from build123d import *

# Parameters (mm, degrees)
F0_W         = 15
F0_H         = 12
F0_R         = 2.5
F1_DEPTH     = 5
F2_R         = 1.5
F3_DEPTH     = 12.001
F4_R         = 0.49999
F5_T1_DEPTH  = 9.5
F5_T3_DEPTH  = 11
F5_T5_DEPTH  = 14
F5_T8_ANGLE  = 90
F5_T10_ANGLE = 90
F5_T12_ANGLE = 90
F5_T14_ANGLE = 90
F5_S17_W     = 0.5
F5_S17_H     = 0.5
F5_T18_DEPTH = 0.5
F5_S23_W     = 0.5
F5_S23_H     = 0.5
F5_T24_DEPTH = 0.5
F5_S29_W     = 0.5
F5_S29_H     = 0.5
F5_T30_DEPTH = 0.5
F5_S35_W     = 0.5
F5_S35_H     = 0.5
F5_T36_DEPTH = 0.5


# Not quite as in the source:
# - a fillet or chamfer that OpenCascade refuses, or shapes differently, is made with other operations: its cross-section is extruded or revolved along the edge and cut away or added
# - a fillet or chamfer is up to 0.001 mm smaller than in the source, because OpenCascade refuses the exact size


with BuildPart() as f1:
    # F0 (on Top) → F1 (new body, symmetric)
    with BuildSketch(Plane.XY):
        with Locations((7.5, 6)):
            Rectangle(F0_W, F0_H)
        with Locations((4.5, 5.5)):
            Circle(F0_R, mode=Mode.SUBTRACT)
    extrude(amount=F1_DEPTH, both=True)

    # F2 (on face) → F3 (cut, through all)
    with BuildSketch(Plane.XZ):
        with Locations((11, 3)):
            Circle(F2_R)
    extrude(amount=-F3_DEPTH, mode=Mode.SUBTRACT)

    # F4 (radius 0.5 in the source; OpenCascade refuses exactly that, so slightly less here)
    f4_edges = [f1.edges().sort_by_distance(p)[0] for p in [
        (7.5, 0, 5),
        (15, 6, 5),
        (7.5, 12, 5),
        (0, 6, 5),
    ]]
    fillet(f4_edges, radius=F4_R)

    # F5: fillet of radius 0.5 on 8 edges, made by hand

    # F5_s2 → F5_t1 (cut)
    with BuildSketch(Plane.XY.offset(-4.5)):
        with BuildLine():
            ThreePointArc((14.5, 0), (14.8535533906, 0.1464466094), (15, 0.5))
            Line((15, 0.5), (15, 0))
            Line((15, 0), (14.5, 0))
        make_face()
        with BuildLine():
            ThreePointArc((0, 0.5), (0.1464466094, 0.1464466094), (0.5, 0))
            Line((0.5, 0), (0, 0))
            Line((0, 0), (0, 0.5))
        make_face()
        with BuildLine():
            ThreePointArc((0, 11.5), (0.1464466094, 11.8535533906), (0.5, 12))
            Line((0.5, 12), (0, 12))
            Line((0, 12), (0, 11.5))
        make_face()
        with BuildLine():
            ThreePointArc((14.5, 12), (14.8535533906, 11.8535533906), (15, 11.5))
            Line((15, 11.5), (15, 12))
            Line((15, 12), (14.5, 12))
        make_face()
    extrude(amount=F5_T1_DEPTH, mode=Mode.SUBTRACT)

    # F5_s4 → F5_t3 (cut)
    with BuildSketch(Plane.XZ.offset(-11.5)):
        with BuildLine():
            ThreePointArc((0, -4.5), (0.1464466094, -4.8535533906), (0.5, -5))
            Line((0.5, -5), (0, -5))
            Line((0, -5), (0, -4.5))
        make_face()
        with BuildLine():
            ThreePointArc((14.5, -5), (14.8535533906, -4.8535533906), (15, -4.5))
            Line((15, -4.5), (15, -5))
            Line((15, -5), (14.5, -5))
        make_face()
    extrude(amount=F5_T3_DEPTH, mode=Mode.SUBTRACT)

    # F5_s6 → F5_t5 (cut)
    with BuildSketch(Plane.YZ.offset(0.5)):
        with BuildLine():
            ThreePointArc((11.5, -5), (11.8535533906, -4.8535533906), (12, -4.5))
            Line((12, -4.5), (12, -5))
            Line((12, -5), (11.5, -5))
        make_face()
        with BuildLine():
            ThreePointArc((0, -4.5), (0.1464466094, -4.8535533906), (0.5, -5))
            Line((0.5, -5), (0, -5))
            Line((0, -5), (0, -4.5))
        make_face()
    extrude(amount=F5_T5_DEPTH, mode=Mode.SUBTRACT)

    # F5_s7 → F5_t8 (revolve, cut)
    with BuildSketch(Plane.XZ.offset(-11.5)):
        with BuildLine():
            ThreePointArc((14.50001, 5), (14.8535563195, 4.8535563195), (15, 4.50001))
            Line((15, 4.50001), (15, 5))
            Line((15, 5), (14.50001, 5))
        make_face()
    revolve(axis=Axis((14.5, 11.5, 5), (0, 0, 1)), revolution_arc=F5_T8_ANGLE, mode=Mode.SUBTRACT)

    # F5_s9 → F5_t10 (revolve, cut)
    with BuildSketch(Plane.YZ.offset(0.5)):
        with BuildLine():
            ThreePointArc((11.50001, 5), (11.8535563195, 4.8535563195), (12, 4.50001))
            Line((12, 4.50001), (12, 5))
            Line((12, 5), (11.50001, 5))
        make_face()
    revolve(axis=Axis((0.5, 11.5, 5), (0, 0, 1)), revolution_arc=F5_T10_ANGLE, mode=Mode.SUBTRACT)

    # F5_s11 → F5_t12 (revolve, cut)
    with BuildSketch(Plane.XZ.offset(-0.5)):
        with BuildLine():
            ThreePointArc((0.49999, 5), (0.1464436805, 4.8535563195), (0, 4.50001))
            Line((0, 4.50001), (0, 5))
            Line((0, 5), (0.49999, 5))
        make_face()
    revolve(axis=Axis((0.5, 0.5, 5), (0, 0, 1)), revolution_arc=F5_T12_ANGLE, mode=Mode.SUBTRACT)

    # F5_s13 → F5_t14 (revolve, cut)
    with BuildSketch(Plane.YZ.offset(14.5)):
        with BuildLine():
            ThreePointArc((0.49999, 5), (0.1464436805, 4.8535563195), (0, 4.50001))
            Line((0, 4.50001), (0, 5))
            Line((0, 5), (0.49999, 5))
        make_face()
    revolve(axis=Axis((14.5, 0.5, 5), (0, 0, 1)), revolution_arc=F5_T14_ANGLE, mode=Mode.SUBTRACT)


with BuildPart() as f5_tool16:
    # F5_s17 → F5_t18 (new body)
    with BuildSketch(Plane.XZ.offset(-0.5)):
        with Locations((14.75, -4.75)):
            Rectangle(F5_S17_W, F5_S17_H)
    extrude(amount=F5_T18_DEPTH)

    # F5_s19 → F5_t20 (revolve, cut)
    with BuildSketch(Plane(origin=(14.5, 0.5, -4.5), x_dir=(-0.7071067812, 0, 0.7071067812), z_dir=(0.7071067812, 0, 0.7071067812))):
        with BuildLine():
            ThreePointArc((0, -0.5), (0.5, 0), (0, 0.5))
            Line((0, 0.5), (0, -0.5))
        make_face()
    revolve(axis=Axis((14.5, 0.5, -4.5), (0, -1, 0)), mode=Mode.SUBTRACT)


with BuildPart() as f1_1:
    add(f1.part)

    # F5_t15: cut F5_tool16
    add(f5_tool16.part, mode=Mode.SUBTRACT)


with BuildPart() as f5_tool22:
    # F5_s23 → F5_t24 (new body)
    with BuildSketch(Plane.YZ.offset(0.5)):
        with Locations((0.25, -4.75)):
            Rectangle(F5_S23_W, F5_S23_H)
    extrude(amount=-F5_T24_DEPTH)

    # F5_s25 → F5_t26 (revolve, cut)
    with BuildSketch(Plane(origin=(0.5, 0.5, -4.5), x_dir=(0, 0.7071067812, 0.7071067812), z_dir=(0, -0.7071067812, 0.7071067812))):
        with BuildLine():
            ThreePointArc((0, -0.5), (0.5, 0), (0, 0.5))
            Line((0, 0.5), (0, -0.5))
        make_face()
    revolve(axis=Axis((0.5, 0.5, -4.5), (-1, 0, 0)), mode=Mode.SUBTRACT)


with BuildPart() as f1_2:
    add(f1_1.part)

    # F5_t21: cut F5_tool22
    add(f5_tool22.part, mode=Mode.SUBTRACT)


with BuildPart() as f5_tool28:
    # F5_s29 → F5_t30 (new body)
    with BuildSketch(Plane.YZ.offset(0.5)):
        with Locations((11.75, -4.75)):
            Rectangle(F5_S29_W, F5_S29_H)
    extrude(amount=-F5_T30_DEPTH)

    # F5_s31 → F5_t32 (revolve, cut)
    with BuildSketch(Plane(origin=(0.5, 11.5, -4.5), x_dir=(0, -0.7071067812, 0.7071067812), z_dir=(0, -0.7071067812, -0.7071067812))):
        with BuildLine():
            ThreePointArc((0, -0.5), (0.5, 0), (0, 0.5))
            Line((0, 0.5), (0, -0.5))
        make_face()
    revolve(axis=Axis((0.5, 11.5, -4.5), (-1, 0, 0)), mode=Mode.SUBTRACT)


with BuildPart() as f1_3:
    add(f1_2.part)

    # F5_t27: cut F5_tool28
    add(f5_tool28.part, mode=Mode.SUBTRACT)


with BuildPart() as f5_tool34:
    # F5_s35 → F5_t36 (new body)
    with BuildSketch(Plane.XY.offset(-4.5)):
        with Locations((14.75, 11.75)):
            Rectangle(F5_S35_W, F5_S35_H)
    extrude(amount=-F5_T36_DEPTH)

    # F5_s37 → F5_t38 (revolve, cut)
    with BuildSketch(Plane(origin=(14.5, 11.5, -4.5), x_dir=(-0.7071067812, -0.7071067812, 0), z_dir=(0.7071067812, -0.7071067812, 0))):
        with BuildLine():
            ThreePointArc((0, -0.5), (0.5, 0), (0, 0.5))
            Line((0, 0.5), (0, -0.5))
        make_face()
    revolve(axis=Axis((14.5, 11.5, -4.5), (0, 0, -1)), mode=Mode.SUBTRACT)


with BuildPart() as f1_4:
    add(f1_3.part)

    # F5_t33: cut F5_tool34
    add(f5_tool34.part, mode=Mode.SUBTRACT)


solid = f1_4.part
The model under review builds one solid part; all positions refer to its coordinate system, in mm. Give positions to 0.01 mm unless a question says otherwise; leave off trailing zeros. Loops run counter-clockwise (first coordinate to the right, second up) from the corner with the lowest first, then second, coordinate; pieces in that order, holes last. Notation, with made-up numbers: (70.5, 10) -> (119.5, 10) arc R11 cw to (119.5, 19) -> close; hole circle Ø3 at (23.5, -21.75). An arc over 180 degrees is marked (long way). Put each result on its own line as item: value. Start each with the question number.
1. We need section C-C on z = 2.25. State the section outline as (x, y) points, then the cut area to 3 significant figures.
2. Mouldability with a two-part tool opening along X and no side actions: class faces 1 (the face through (15, 6, 0)), 2 (the face through (9.8, 5.9, 2.1)), 3 (the face through (7, 0, 0)) as released by +X, released by -X, zero draft, split by the parting line, or undercut.
3. Wall thickness on probe 1 along Y at (x, z) = (4.5, -1); probe 2 along X at (y, z) = (3.75, 4); probe 3 along X at (y, z) = (7, 4): over which ranges is each line inside the solid? List them lowest first.
4. We need section A-A on y = 7. State the section outline as (x, z) points, then the cut area to 3 significant figures.
5. We need section D-D on z = -2.25. State the section outline as (x, y) points, then the cut area to 3 significant figures.
Determined:
1. outline: (0, 0.5) arc R0.5 ccw to (0.5, 0) -> (9.7, 0) -> (9.7, 12) -> (0.5, 12) arc R0.5 ccw to (0, 11.5) -> close; (12.3, 0) -> (14.5, 0) arc R0.5 ccw to (15, 0.5) -> (15, 11.5) arc R0.5 ccw to (14.5, 12) -> (12.3, 12) -> close; hole circle Ø5 at (4.5, 5.5)
1. area: 129 mm^2
2. face 1: released by +X
2. face 2: undercut
2. face 3: zero draft
3. probe 1: 0 to 3, 8 to 12
3. probe 2: 0 to 2.71, 6.29 to 9.88, 12.12 to 15
3. probe 3: 0 to 2.5, 6.5 to 9.88, 12.12 to 15
4. outline: (0, -4.5) arc R0.5 ccw to (0.5, -5) -> (2.5, -5) -> (2.5, 5) -> (0.5, 5) arc R0.5 ccw to (0, 4.5) -> close; (6.5, -5) -> (14.5, -5) arc R0.5 ccw to (15, -4.5) -> (15, 4.5) arc R0.5 ccw to (14.5, 5) -> (6.5, 5) -> close; hole circle Ø3 at (11, 3)
4. area: 103 mm^2
5. outline: (0, 0.5) arc R0.5 ccw to (0.5, 0) -> (14.5, 0) arc R0.5 ccw to (15, 0.5) -> (15, 11.5) arc R0.5 ccw to (14.5, 12) -> (0.5, 12) arc R0.5 ccw to (0, 11.5) -> close; hole circle Ø5 at (4.5, 5.5)
5. area: 160 mm^2
